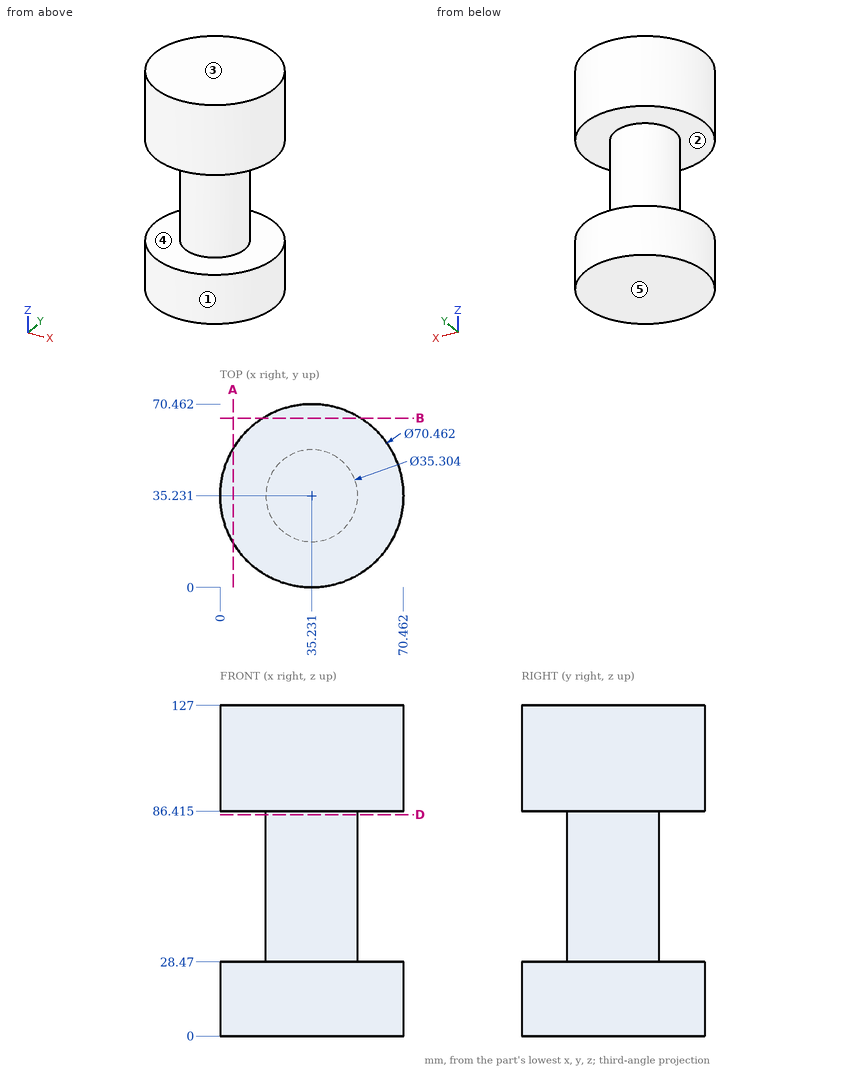
Answer from the drawing. Dimensions are ordinates in mm from the lowest x, y and z of the part. A direction names the side the tool comes from. Give positions to 0.01 mm unless a question says otherwise; leave off trailing zeros. Loops run counter-clockwise (first coordinate to the right, second up) from the corner with the lowest first, then second, coordinate; pieces in that order, holes last. Notation, with made-up numbers: (27, 21) -> (61, 21) arc R23 cw to (61, 37) -> close; hole circle Ø6 at (86.25, 54.25). An arc over 180 degrees is marked (long way). One line per question, with ' | ' between items. Start each with the question number.
1) Section B-B, the plane y = 65 is taken. Determine the outline of the cut face in (x, z) (1 decimal), then the cut area to 3 significant figures.
2) Determine the mould class of the marked faces 3, 4 and 5 for opening direction Z: +Z half, -Z half, draft (parallel to the pull), parting line (faces both ways), or undercut.
3) For the marked faces 1 and 2, determine the directions among +Z, -Z, +X, -X, +Y, -Y from which every point of the face is accessible in a straight line to the end or side of a thin tool.
4) Straight lines are drawn through the part: L1, parallel to Z at x = 36, y = 55 (1 decimal); L2, parallel to Y at x = 36, z = 114.5 (1 decimal); L3, parallel to X at y = 19.5, z = 117 (1 decimal). For each, find the intervals that lie inside material, in ascending order.
5) Section A-A, the plane x = 5 is taken. Determine the outline of the cut face in (y, z) (1 decimal), then the cut area to 3 significant figures.
6) Each of these flat-tipped pins is pushed along its axis until it touches: pin 1 (1 mm diameter, centred on x = 29.5, y = 15, fed in from -Z); pin 2 (1.5 mm diameter, centred on y = 23, z = 55, fed in from -X); pin 3 (8 mm diameter, centred on x = 21, z = 33, fed in from -Y); pin 4 (10 mm diameter, centred on y = 52.5, z = 34, fed in from -X). Where does it stop, or does it pass through?
7) Section D-D, the plane z = 85 is taken. Determine the outline of the cut face in (x, y) (1 decimal), then the cut area to 3 significant figures.
Resolved:
1) outline: (16.4, 0) -> (54.1, 0) -> (54.1, 28.5) -> (16.4, 28.5) -> close; (16.4, 86.4) -> (54.1, 86.4) -> (54.1, 127) -> (16.4, 127) -> close | area: 2,600 mm2
2) face 3: +Z half | face 4: undercut | face 5: -Z half
3) face 1: +Z, -Z | face 2: none
4) L1: 0 to 28.5, 86.4 to 127 | L2: 0 to 70.5 | L3: 3.7 to 66.8
5) outline: (17.1, 0) -> (53.3, 0) -> (53.3, 28.5) -> (17.1, 28.5) -> close; (17.1, 86.4) -> (53.3, 86.4) -> (53.3, 127) -> (17.1, 127) -> close | area: 2,500 mm2
6) pin 1: z = 0 | pin 2: x = 21.82 | pin 3: y = 20.85 | pin 4: x = 22.54
7) outline: circle Ø35.3 at (35.2, 35.2) | area: 979 mm2
